Part model, mm, in its own coordinate system. Face numbers are marked on the shaded views. A direction names the side the tool comes from. Round coordinates to 2 decimals unless told otherwise and drop trailing zeros. Loops run counter-clockwise (first coordinate to the right, second up) from the corner with the lowest first, then second, coordinate; pieces in that order, holes last. Notation, with made-up numbers: M -15.5,62 L -11.5,62 A7 ccw -11.5,67 Z; hole C 65.25,-5.75 d7. An arc over 180 degrees is marked long. Write each question's results on one line, items separated by ' | '.
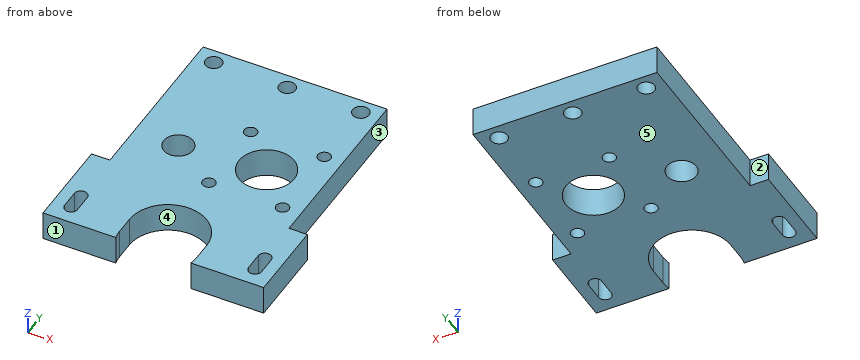
Autodesk Inventor part; units mm, degrees
ref_plane "YZ Plane" through (0, 0, 0) normal (1, 0, 0) x (0, 1, 0)
ref_plane "XZ Plane" through (0, 0, 0) normal (0, 1, 0) x (-1, 0, 0)
ref_plane "XY Plane" through (0, 0, 0) normal (0, 0, 1) x (1, 0, 0)
sketch "Sketch1" plane through (0, 0, 0) normal (0, 0, 1) x (1, 0, 0)
  line L0 (-30, 32.5) -> (30, 32.5)
  line L1 (30, 32.5) -> (30, -32.5)
  line L2 (30, -32.5) -> (-30, -32.5)
  line L3 (-30, -32.5) -> (-30, 32.5)
  point P0 (0, 0)
  point P1 (0, 32.5)
  point P2 (-30, 0)
  dimension "d0" = 60
  dimension "d1" = 65
extrude "Extrusion1" add sketch "Sketch1" along normal blind 8
sketch "Sketch4" plane through (0, 0, 8) normal (0, 0, 1) x (1, 0, 0)
  circle A0 centre (-25, -15) radius 1.75
  circle A1 centre (25, -15) radius 1.75
  circle A2 centre (25, -25) radius 1.75
  arc A3 (-10.5, -30) -> (10.5, -30) centre (0, -30) ccw
  line L0 (10.5, -30) -> (10.5, -25)
  arc A4 (10.5, -25) -> (-10.5, -25) centre (0, -25) ccw
  line L1 (-10.5, -25) -> (-10.5, -30)
  line L2 (30, -10) -> (30, -50)
  line L3 (30, -50) -> (-30, -50)
  line L4 (-30, -50) -> (-30, -10)
  line L5 (-30, -10) -> (30, -10)
  line L6 (25, -27.5) -> (25, -22.5) construction
  line L7 (26.75, -27.5) -> (26.75, -22.5)
  line L8 (23.25, -22.5) -> (23.25, -27.5)
  arc A5 (23.25, -27.5) -> (26.75, -27.5) centre (25, -27.5) ccw
  arc A6 (26.75, -22.5) -> (23.25, -22.5) centre (25, -22.5) ccw
  line L9 (-25, -27.5) -> (-25, -22.5) construction
  line L10 (-23.25, -27.5) -> (-23.25, -22.5)
  line L11 (-26.75, -22.5) -> (-26.75, -27.5)
  arc A7 (-26.75, -27.5) -> (-23.25, -27.5) centre (-25, -27.5) ccw
  arc A8 (-23.25, -22.5) -> (-26.75, -22.5) centre (-25, -22.5) ccw
  line L12 (-30, -32.5) -> (30, -32.5)
  point P0 (0, 0)
  point P1 (-25, -25)
  point P2 (26.75, -25)
  point P3 (23.25, -25)
  dimension "d22" = 5
  dimension "d23" = 3.5
  dimension "d24" = 5
  dimension "d25" = 10.5
  dimension "d26" = 7.5
  dimension "d27" = 30
extrude "Extrusion4" cut sketch "Sketch4" against normal blind 10 contours A2 | L7 A5 L8 A2 | A2 L8 A6 L7 | L1 A4 L0 A3 L12 | L12 A3 | A7 L11 A8 L10
sketch "Sketch5" plane through (0, 0, 8) normal (0, 0, 1) x (1, 0, 0)
  circle A0 centre (10, 6.8914) radius 7.5
  line L0 (30, 32.5) -> (-30, 32.5)
  line L1 (30, -32.5) -> (30, 32.5)
  point P0 (0, 0)
  dimension "d13" = 15
  dimension "d28" = 25.6086
  dimension "d29" = 20
extrude "Extrusion5" cut sketch "Sketch5" against normal through all
sketch "Sketch6" plane through (0, 0, 8) normal (0, 0, 1) x (1, 0, 0)
  circle A0 centre (20, 17.6414) radius 1.75
  circle A1 centre (0, 17.6414) radius 1.75
  circle A2 centre (0, -3.8586) radius 1.75
  circle A3 centre (20, -3.8586) radius 1.75
  line L0 (0, 17.6414) -> (20, 17.6414) construction
  line L1 (20, 17.6414) -> (20, -3.8586) construction
  line L2 (20, -3.8586) -> (0, -3.8586) construction
  line L3 (0, -3.8586) -> (0, 17.6414) construction
  line L4 (30, -32.5) -> (30, 32.5) construction
  line L5 (30, 32.5) -> (-30, 32.5) construction
  circle A4 centre (10, 6.8914) radius 7.5
  point P0 (0, 0)
  point P1 (10, -3.8586)
  point P2 (20, 6.8914)
  dimension "d31" = 21.5
  dimension "d33" = 3.5
  dimension "d42" = 20
extrude "Extrusion6" cut sketch "Sketch6" against normal through all contours A0 | A1 | A2 | A3
sketch "Sketch7" plane through (0, 0, 8) normal (0, 0, 1) x (1, 0, 0)
  line L0 (-30, 32.5) -> (-30, -32.5)
  line L1 (-30, -7.5) -> (-25, -7.5)
  line L2 (-25, -7.5) -> (-25, 32.5)
  line L3 (-25, 32.5) -> (-30, 32.5)
  line L4 (-30, 32.5) -> (-30, -7.5)
  line L5 (30, 32.5) -> (-30, 32.5)
  line L6 (30, -10) -> (-30, -10)
  line L7 (25, -10) -> (30, -10)
  line L8 (30, -10) -> (30, 32.5)
  line L9 (30, 32.5) -> (25, 32.5)
  line L10 (25, 32.5) -> (25, -10)
  line L11 (30, -32.5) -> (30, 32.5)
  point P0 (0, 0)
  point P1 (25, -10)
  dimension "d18" = 5
  dimension "d19" = 5
  dimension "d43" = 40
extrude "Extrusion7" cut sketch "Sketch7" against normal through all contours L3 L2 L1 L0 | L5 L8 L6 L10
sketch "Sketch8" plane through (0, 0, 8) normal (0, 0, 1) x (1, 0, 0)
  circle A0 centre (-13, 5.0309) radius 4
  line L0 (-30, -7.5) -> (-30, -32.5)
  line L1 (25, 32.5) -> (-25, 32.5)
  point P0 (0, 0)
  dimension "d35" = 8
  dimension "d36" = 17
  dimension "d37" = 27.4691
extrude "Extrusion8" cut sketch "Sketch8" against normal blind 10
move faces "Move1" translate (0, 8, 0) faces at (8.3333, 32.5, 2.6667)
sketch "Sketch9" plane through (0, 0, 0) normal (0, 0, -1) x (-1, 0, 0)
  line L0 (-25, 40.5) -> (25, 40.5)
  point P0 (0, 0)
  point P1 (0, 36.5)
  point P2 (-20, 36.5)
  point P3 (20, 36.5)
  dimension "d47" = 20
  dimension "d48" = 20
  dimension "d49" = 4
hole "Hole1" at (0, 36.5, 0) at (20, 36.5, 0) at (-20, 36.5, 0) direction (0, 0, 1) diameter 4.5 end through all
equation "\"d19\" = d18"
properties part number "0005-10-005"
Item 1: Which spindle directions (+Z, -Z, +X, -X, +Y, -Y) get a long thin tool onto all of the face, cutting with end or side? Do the marked faces 1, 2, 3, 4 and 5. Say none if no direction does.
Filled sheet:
face 1: +Z, -Z, +X, -X, -Y | face 2: +Z, -Z, -X, +Y | face 3: +Z, -Z, +X, +Y | face 4: +Z, -Z | face 5: -Z, +X, -X, +Y, -Y
Item 2: Band-saw the part on D-D on x = -13. Give the cut face in (y, z).
Filled sheet:
outline: M -32.5,0 L 1.03,0 L 1.03,8 L -32.5,8 Z; M 9.03,0 L 40.5,0 L 40.5,8 L 9.03,8 Z
Item 3: Band-saw the part on A-A on x = -20. Give the cut face in (y, z).
Filled sheet:
outline: M -32.5,0 L 34.25,0 L 34.25,8 L -32.5,8 Z; M 38.75,0 L 40.5,0 L 40.5,8 L 38.75,8 Z
Item 4: Band-saw the part on B-B on x = 0. Give the cut face in (y, z), and give its area (3 significant figures).
Filled sheet:
outline: M -14.5,0 L -5.61,0 L -5.61,8 L -14.5,8 Z; M -2.11,0 L 15.89,0 L 15.89,8 L -2.11,8 Z; M 19.39,0 L 34.25,0 L 34.25,8 L 19.39,8 Z; M 38.75,0 L 40.5,0 L 40.5,8 L 38.75,8 Z | area: 348 mm^2
Item 5: Drop flat-ended pins along their axis: P1, Ø8, axis at x = 11, y = -10.5, coming from the -Z side; P2, Ø2.5, axis at x = 0, y = 36.5, coming from the +Z side; P3, Ø1.5, axis at x = 28.5, z = 4.5, coming from the +Y side; P4, Ø1.5, axis at x = -26.5, z = 2.5, coming from the +Y side. Give the stop position or say it passes through.
Filled sheet:
P1: z = 0 | P2: through | P3: y = -10 | P4: y = -7.5
Item 6: Wall check: L1, parallel to Y at x = 20, z = 3; L2, parallel to X at y = -22, z = 7.25; L3, parallel to X at y = -28, z = 5.75. Give the ranges that are in metal, low to high.
Filled sheet:
L1: -32.5 to -5.61, -2.11 to 15.89, 19.39 to 34.25, 38.75 to 40.5 | L2: -30 to -26.68, -23.32 to -10.06, 10.06 to 23.32, 26.68 to 30 | L3: -30 to -26.68, -23.32 to -10.5, 10.5 to 23.32, 26.68 to 30
Item 7: Band-saw the part on C-C on z = 2.5. Count the separate pieces of the cut face and the enclosed holes in it, and give its area (3 significant figures).
Filled sheet:
separate pieces: 1 | enclosed holes: 11 | area: 3,190 mm^2
